```python
from build123d import *

# Parameters (mm, degrees)
F0_W     = 77.2405713797
F0_H     = 77.8463184834
F0_R     = 17.1685214952
F1_DEPTH = 50.8
F2_R     = 5.08
F3_R     = 13.396248622
F4_DEPTH = 228.6


with BuildPart() as f1:
    # F0 (on Front) → F1 (new body)
    with BuildSketch(Plane.XZ):
        with Locations((-2.95496732, -1.6224384308)):
            Rectangle(F0_W, F0_H)
        Circle(F0_R, mode=Mode.SUBTRACT)
    extrude(amount=F1_DEPTH)

    # F2
    f2_edges = [f1.edges().sort_by_distance(p)[0] for p in [
        (-2.954967, -50.8, -40.545598),
        (35.665318, -50.8, -1.622438),
        (-2.954967, -50.8, 37.300721),
        (-41.575253, -50.8, -1.622438),
        (-17.168521, -50.8, 0),
    ]]
    fillet(f2_edges, radius=F2_R)

    # F3 (on face) → F4 (cut)
    with BuildSketch(Plane(origin=(0, 0, -40.5455976725), x_dir=(1, 0, 0), z_dir=(0, 0, -1))):
        with Locations((0, 28.7160556763)):
            Circle(F3_R)
    extrude(amount=-F4_DEPTH, mode=Mode.SUBTRACT)


solid = f1.part
```
Source: CAD feature listing. Evaluate the final solid. Frame: model axes, mm. Give positions to 0.01 mm unless a question says otherwise; leave off trailing zeros. Write each loop counter-clockwise with the first axis right and the second up, starting at its lowest first coordinate (ties: lowest second). Pieces come first, ordered by that corner, then holes.
1. Section query A-A (z = 0). Return the cut outline in (x, y).
2. Material intervals for line 1 along Z through (x, y) = (0, -11.5); line 2 along Y through (x, z) = (0.5, -23.5); line 3 along Y through (x, z) = (-10.5, 23.5), sorted ascending.
3. First-contact query: pin 1 (1 mm diameter, centred on x = 17, z = -10, fed in from -Y). Flat tip, straight axial feed; report the tip coordinate or a pass-through.
4. Pull-direction query (Y, two-part tool) for faces 1 (the face through (7.202, -40.012, -25.85)), 2 (the face through (35.665, -23, -2)), 3 (the face through (-21, 0, -1)); classes: +Y half, -Y half, draft (parallel to the pull), parting line (faces both ways), or undercut.
5. Section query C-C (y = -25). Return the cut outline in (x, z), then the cut area to 3 significant figures.
6. Section query B-B (x = 0). Return the cut outline in (y, z).
7. Section query D-D (y = -11). Return the cut outline in (x, z), then the cut area to 3 significant figures.
Output values:
1. outline: (-41.58, -45.72) arc R5.08 ccw to (-36.5, -50.8) - (-22.25, -50.8) arc R5.08 ccw to (-17.17, -45.72) - (-17.17, 0) - (-41.58, 0) - close; (17.17, -45.72) arc R5.08 ccw to (22.25, -50.8) - (30.59, -50.8) arc R5.08 ccw to (35.67, -45.72) - (35.67, 0) - (17.17, 0) - close
2. line 1: z = -40.55 to -17.17, 17.17 to 37.3
2. line 2: y = -50.8 to -42.1, -15.33 to 0
2. line 3: y = -50.8 to -37.04, -20.4 to 0
3. pin 1: stops at y = -50.38
4. face 1: undercut
4. face 2: draft
4. face 3: +Y half
5. outline: (-41.58, -40.55) - (-12.87, -40.55) - (-12.87, -11.36) arc R17.17 cw to (-12.87, 11.36) - (-12.87, 37.3) - (-41.58, 37.3) - close; (12.87, -40.55) - (35.67, -40.55) - (35.67, 37.3) - (12.87, 37.3) - (12.87, 11.36) arc R17.17 cw to (12.87, -11.36) - close
5. area: 3,880 mm2
6. outline: (-50.8, -35.47) arc R5.08 ccw to (-45.72, -40.55) - (-42.11, -40.55) - (-42.11, -17.17) - (-45.72, -17.17) arc R5.08 ccw to (-50.8, -22.25) - close; (-50.8, 22.25) arc R5.08 ccw to (-45.72, 17.17) - (-42.11, 17.17) - (-42.11, 37.3) - (-45.72, 37.3) arc R5.08 ccw to (-50.8, 32.22) - close; (-15.32, -40.55) - (0, -40.55) - (0, -17.17) - (-15.32, -17.17) - close; (-15.32, 17.17) - (0, 17.17) - (0, 37.3) - (-15.32, 37.3) - close
7. outline: (-41.58, -40.55) - (35.67, -40.55) - (35.67, 37.3) - (-41.58, 37.3) - close; hole circle Ø34.34 at (0, 0)
7. area: 5,090 mm2
